Check sheet for the modelled part. Datum: model origin and axes. Units: mm. A direction names the side the tool comes from. Give positions to 0.01 mm unless a question says otherwise; leave off trailing zeros. Loops run counter-clockwise (first coordinate to the right, second up) from the corner with the lowest first, then second, coordinate; pieces in that order, holes last. Notation, with made-up numbers: M -9,68 L 9,68 A16 cw 9,79 Z; hole C 52,69.5 d8. An arc over 180 degrees is marked long. Write each question's results on one line, items separated by ' | '. Start each with the question number.
1. Draft check along Y on faces 6 (the cylindrical face through (30, 101, -1)), 7 (the flat face through (-1, 0, -49)), 8 (the cylindrical face through (43, 2, -89)). Enter one of: pulls with the +Y half, pulls with the -Y half, needs draft (parallel to the pull), parting line crosses it, or undercut.
2. Sectioned sample at D-D on x = 3. Record the cut outline in (y, z), and give its area (3 significant figures).
3. Material ranges on line 1 along X through (y, z) = (1.25, -83); line 2 along Z through (x, y) = (36, 61.5); line 3 along Y through (x, z) = (37.5, -25.5), recorded low to high.
4. Sectioned sample at A-A on z = -69. Record the cut outline in (x, y).
5. Sectioned sample at C-C on y = 88. Record the cut outline in (x, z).
6. Sectioned sample at B-B on y = 25.5. Record the cut outline in (x, z), and give its area (3 significant figures).
7. Go/stop test with flat-tipped pins: pin 1 (1 mm diameter, centred on x = -11, z = -70.5, fed in from +Y); pin 2 (4 mm diameter, centred on x = 15, z = -69, fed in from -Y); pin 3 (3.5 mm diameter, centred on x = -6, y = 1, fed in from +Z). Record where each tip stops, or that it passes through.
8. Tool access check on faces 1 (the cylindrical face through (30, 79, -1)), 2 (the flat face through (1, 1, -90)), 3 (the flat face through (-1, 65, -3)), 4 (the flat face through (-20, 15, -2)), 5 (the flat face through (0, 2, -10)). Record the directions out of +Z, -Z, +X, -X, +Y, -Y that give a thin tool (end or side, any length) a straight path to the whole face; none if there is none.
```python
from build123d import *

# Parameters (mm, degrees)
BOSS_EXTRUDE1_DEPTH        = 45
FLATTEN_BENDS1_START       = -45
FLATTEN_BENDS1_OUTLINE_W   = 122
FLATTEN_BENDS1_OUTLINE_H   = 3
FLATTEN_BENDS1_DEPTH       = 90
FLATTEN_BENDS1_2_OUTLINE_W = 3
FLATTEN_BENDS1_2_OUTLINE_H = 119.533030317
FLATTEN_BENDS1_2_DEPTH     = 90
PROCESS_BENDS1_START       = -45
PROCESS_BENDS1_DEPTH       = 90
PROCESS_BENDS1_2_DEPTH     = 90
SKETCH8_W                  = 40
SKETCH8_H                  = 6.6
SKETCH8_H_2                = 23.4
CUT_EXTRUDE1_DEPTH         = 10
FILLET1_R                  = 3
FILLET2_R                  = 5
CUT_EXTRUDE2_DEPTH         = 80
SKETCH10_R                 = 2.1
CUT_EXTRUDE3_DEPTH         = 80


# Read off the part's stored shape, not the designer's step: Flatten-Bends1, Process-Bends1
with BuildPart() as part:
    # Sketch1 → Boss-Extrude1 (new, symmetric)
    with BuildSketch(Plane(origin=(0, 0, 0), x_dir=(0, 0, -1), z_dir=(1, 0, 0))):
        Polygon((0, 125), (0, 0), (90, 0), (90, 3), (3, 3), (3, 125), align=None)
    extrude(amount=BOSS_EXTRUDE1_DEPTH, both=True)

    # Flatten-Bends1 outline → Flatten-Bends1 (cut)
    with BuildSketch(Plane.YZ.offset(FLATTEN_BENDS1_START)):
        with Locations((64, -1.5)):
            Rectangle(FLATTEN_BENDS1_OUTLINE_W, FLATTEN_BENDS1_OUTLINE_H)
    extrude(amount=FLATTEN_BENDS1_DEPTH, mode=Mode.SUBTRACT)

    # Flatten-Bends1 2 outline → Flatten-Bends1 2 (add)
    with BuildSketch(Plane.YZ.offset(FLATTEN_BENDS1_START)):
        with Locations((1.5, 59.766515159)):
            Rectangle(FLATTEN_BENDS1_2_OUTLINE_W, FLATTEN_BENDS1_2_OUTLINE_H)
    extrude(amount=FLATTEN_BENDS1_2_DEPTH)

    # Process-Bends1 outline → Process-Bends1 (cut)
    with BuildSketch(Plane.YZ.offset(PROCESS_BENDS1_START)):
        with BuildLine():
            ThreePointArc((0, -6.6), (0.798276118, -3.453573455), (3, -1.068273325))
            Line((3, -1.068273325), (3, 119.533030317))
            Line((3, 119.533030317), (0, 119.533030317))
            Line((0, 119.533030317), (0, -6.6))
        make_face()
    extrude(amount=PROCESS_BENDS1_DEPTH, mode=Mode.SUBTRACT)

    # Process-Bends1 2 outline → Process-Bends1 2 (add)
    with BuildSketch(Plane.YZ.offset(PROCESS_BENDS1_START)):
        with BuildLine():
            Line((6.6, -3), (125, -3))
            Line((125, -3), (125, 0))
            Line((125, 0), (6.6, 0))
            ThreePointArc((6.6, 0), (4.722421247, -0.272702154), (3, -1.068273325))
            Line((3, -1.068273325), (3, -6.6))
            ThreePointArc((3, -6.6), (4.054415588, -4.054415588), (6.6, -3))
        make_face()
    extrude(amount=PROCESS_BENDS1_2_DEPTH)

    # Sketch8 → Cut-Extrude1 (cut)
    with BuildSketch(Plane.XY):
        with BuildLine():
            ThreePointArc((-20, 30), (0, 50), (20, 30))
            Line((20, 30), (-20, 30))
        make_face()
        with Locations((0, 3.3)):
            Rectangle(SKETCH8_W, SKETCH8_H)
        with Locations((0, 18.3)):
            Rectangle(SKETCH8_W, SKETCH8_H_2)
    extrude(amount=-CUT_EXTRUDE1_DEPTH, mode=Mode.SUBTRACT)

    # Fillet1
    fillet1_edges = [part.edges().sort_by_distance(p)[0] for p in [
        (-20, 1.5, -10),
        (20, 1.5, -10),
    ]]
    fillet(fillet1_edges, radius=FILLET1_R)

    # Fillet2
    fillet2_edges = [part.edges().sort_by_distance(p)[0] for p in [
        (-45, 125, -1.5),
        (45, 125, -1.5),
        (45, 1.5, -90),
        (-45, 1.5, -90),
    ]]
    fillet(fillet2_edges, radius=FILLET2_R)

    # Sketch9 → Cut-Extrude2 (cut)
    with BuildSketch(Plane.XY):
        with BuildLine():
            Line((-26.5, 97.5), (-26.5, 82.5))
            ThreePointArc((-26.5, 82.5), (-30, 79), (-33.5, 82.5))
            Line((-33.5, 82.5), (-33.5, 97.5))
            ThreePointArc((-33.5, 97.5), (-30, 101), (-26.5, 97.5))
        make_face()
        with BuildLine():
            Line((26.5, 97.5), (26.5, 82.5))
            ThreePointArc((26.5, 82.5), (30, 79), (33.5, 82.5))
            Line((33.5, 82.5), (33.5, 97.5))
            ThreePointArc((33.5, 97.5), (30, 101), (26.5, 97.5))
        make_face()
    extrude(amount=-CUT_EXTRUDE2_DEPTH, mode=Mode.SUBTRACT)

    # Sketch10 → Cut-Extrude3 (cut)
    with BuildSketch(Plane(origin=(0, 3, 0), x_dir=(1, 0, 0), z_dir=(0, 1, 0))):
        with Locations(Location((-10, 83, 0), (0, 0, 270))):
            Circle(SKETCH10_R)
        with Locations(Location((10, 83, 0), (0, 0, 270))):
            Circle(SKETCH10_R)
        with Locations(Location((-15, 69, 0), (0, 0, 270))):
            Circle(SKETCH10_R)
        with Locations(Location((15, 69, 0), (0, 0, 270))):
            Circle(SKETCH10_R)
    extrude(amount=-CUT_EXTRUDE3_DEPTH, mode=Mode.SUBTRACT)


solid = part.part
```
Output values:
1) face 6: undercut | face 7: pulls with the -Y half | face 8: needs draft
2) outline: M 0,-90 L 3,-90 L 3,-10 L 0,-10 Z; M 49.77,-3 L 125,-3 L 125,0 L 49.77,0 Z | area: 466 mm2
3) line 1: -45 to -12.1, -7.9 to 7.9, 12.1 to 45 | line 2: -3 to 0 | line 3: 0 to 3
4) outline: M -45,0 L -17.1,0 L -17.1,3 L -45,3 Z; M -12.9,0 L 12.9,0 L 12.9,3 L -12.9,3 Z; M 17.1,0 L 45,0 L 45,3 L 17.1,3 Z
5) outline: M -45,-3 L -33.5,-3 L -33.5,0 L -45,0 Z; M -26.5,-3 L 26.5,-3 L 26.5,0 L -26.5,0 Z; M 33.5,-3 L 45,-3 L 45,0 L 33.5,0 Z
6) outline: M -45,-3 L -20,-3 L -20,0 L -45,0 Z; M 20,-3 L 45,-3 L 45,0 L 20,0 Z | area: 150 mm2
7) pin 1: y = 3 | pin 2: through | pin 3: z = -10
8) face 1: +Z, -Z | face 2: -Z, +X, -X, +Y, -Y | face 3: -Z, +X, -X, +Y | face 4: +Z, -Y | face 5: +Z, +Y, -Y
